```python
from build123d import *

# Parameters (mm, degrees)
F0_W     = 25.4
F0_H     = 25.4
F0_R     = 2.6035
F1_DEPTH = 12.5
F3_DEPTH = 25.001


with BuildPart() as f1:
    # F0 (on Front) → F1 (new body, symmetric)
    with BuildSketch(Plane.XZ):
        Rectangle(F0_W, F0_H)
        Circle(F0_R, mode=Mode.SUBTRACT)
    extrude(amount=F1_DEPTH, both=True)

    # F2 (on face) → F3 (cut, through all)
    with BuildSketch(Plane.XZ.offset(12.5)):
        Polygon((3.2385, 12.7), (-3.2385, 12.7), (-3.2385, 10.4902), (-7.4295, 10.4902), (-1.4478, 4.5085), (1.4478, 4.5085), (7.4295, 10.4902), (3.2385, 10.4902), align=None)
        Polygon((-12.7, 3.2385), (-12.7, -3.2385), (-10.4902, -3.2385), (-10.4902, -7.4295), (-4.5085, -1.4478), (-4.5085, 1.4478), (-10.4902, 7.4295), (-10.4902, 3.2385), align=None)
        Polygon((-3.2385, -12.7), (3.2385, -12.7), (3.2385, -10.4902), (7.4295, -10.4902), (1.4478, -4.5085), (-1.4478, -4.5085), (-7.4295, -10.4902), (-3.2385, -10.4902), align=None)
        Polygon((12.7, -3.2385), (12.7, 3.2385), (10.4902, 3.2385), (10.4902, 7.4295), (4.5085, 1.4478), (4.5085, -1.4478), (10.4902, -7.4295), (10.4902, -3.2385), align=None)
    extrude(amount=-F3_DEPTH, mode=Mode.SUBTRACT)


solid = f1.part
```
The listing builds one solid part. Answer for the finished solid, in the listing's coordinates (mm). A direction names the side the tool comes from. Coordinates: 2 decimals unless noted, no trailing zeros. Loops run counter-clockwise (first coordinate to the right, second up) from the corner with the lowest first, then second, coordinate; pieces in that order, holes last. Notation, with made-up numbers: M 31,15.25 L 64,15.25 A29 ccw 64,50.25 Z; hole C 53,86 d10. An arc over 180 degrees is marked long. Answer as a JSON object with one key per item and string values. Group by question number.
Item 1: Each of these flat-tipped pins is pushed along its axis until it touches: P1, Ø1, axis at x = -8, z = -3.5, coming from the +Y side; P2, Ø1.5, axis at y = 10, z = 0, coming from the +X side; P3, Ø1.4, axis at x = 0, y = -5, coming from the -Z side; P4, Ø2.5, axis at y = 2.5, z = 0, coming from the -X side. Where does it stop, or does it pass through?
Item 2: Section B-B (x = 0) is taken. Write down the section's boundary in (y, z), and give its area (4 significant figures).
Item 3: Consider L1, parallel to Z at x = 0, y = 7.5; L2, parallel to X at y = -0.25, z = 5.5; L3, parallel to Z at x = -6.25, y = 1.5. Determine where each line is inside the solid, lowest interval first.
Item 4: Which of the six approach directions +Z, -Z, +X, -X, +Y, -Y give full straight-line access (tool end or side, diameter ignored) to faces 4 (the face through (-3.238, 0, -12)), 5 (the face through (-7.54, -0.17, -4.48)), 6 (the face through (-12, 0, 3.238)), 7 (the face through (4.508, 0, 0))?
Item 5: Section A-A (z = 0) is taken. Write down the section's boundary in (x, y).
Item 6: Section C-C (z = 5.25) is taken. Write down the section's boundary in (x, y).
Item 7: Determine the mould class of faces 1 (the face through (-10.49, 0, -5)), 2 (the face through (8, 0, -12.7)), 3 (the face through (3, -12.5, 0)) for opening direction Z: +Z half, -Z half, draft (parallel to the pull), parting line (faces both ways), or undercut.
Solved:
{
 "1": {"P1": "passes through", "P2": "stops at x = 4.51", "P3": "stops at z = -4.51", "P4": "stops at x = -4.51"},
 "2": {"outline": "M -12.5,-4.51 L 12.5,-4.51 L 12.5,-2.6 L -12.5,-2.6 Z; M -12.5,2.6 L 12.5,2.6 L 12.5,4.51 L -12.5,4.51 Z", "area": "95.25 mm2"},
 "3": {"L1": "z = -4.51 to -2.6, 2.6 to 4.51", "L2": "x = -12.7 to -10.49, -8.56 to -2.44, 2.44 to 8.56, 10.49 to 12.7", "L3": "z = -12.7 to -10.49, -9.31 to -3.19, 3.19 to 9.31, 10.49 to 12.7"},
 "4": {"face 4": "-Z, +Y, -Y", "face 5": "+Y, -Y", "face 6": "-X, +Y, -Y", "face 7": "+X, +Y, -Y"},
 "5": {"outline": "M -4.51,-12.5 L -2.6,-12.5 L -2.6,12.5 L -4.51,12.5 Z; M 2.6,-12.5 L 4.51,-12.5 L 4.51,12.5 L 2.6,12.5 Z"},
 "6": {"outline": "M -12.7,-12.5 L -10.49,-12.5 L -10.49,12.5 L -12.7,12.5 Z; M -8.31,-12.5 L -2.19,-12.5 L -2.19,12.5 L -8.31,12.5 Z; M 2.19,-12.5 L 8.31,-12.5 L 8.31,12.5 L 2.19,12.5 Z; M 10.49,-12.5 L 12.7,-12.5 L 12.7,12.5 L 10.49,12.5 Z"},
 "7": {"face 1": "undercut", "face 2": "-Z half", "face 3": "draft"}
}
